Here's the drawing with two shaded views (mm, measured from the low corner). I have some questions. Give positions to 0.01 mm unless a question says otherwise; leave off trailing zeros. Write each loop counter-clockwise with the first axis right and the second up, starting at its lowest first coordinate (ties: lowest second). Pieces come first, ordered by that corner, then holes. Notation, with made-up numbers: (56, 31.5) - (98, 31.5) arc R21 cw to (98, 70.5) - close; hole circle Ø5 at (-34.5, 61.5). An arc over 180 degrees is marked (long way). Answer as a JSON object with one key per item and string values. Group by question number.
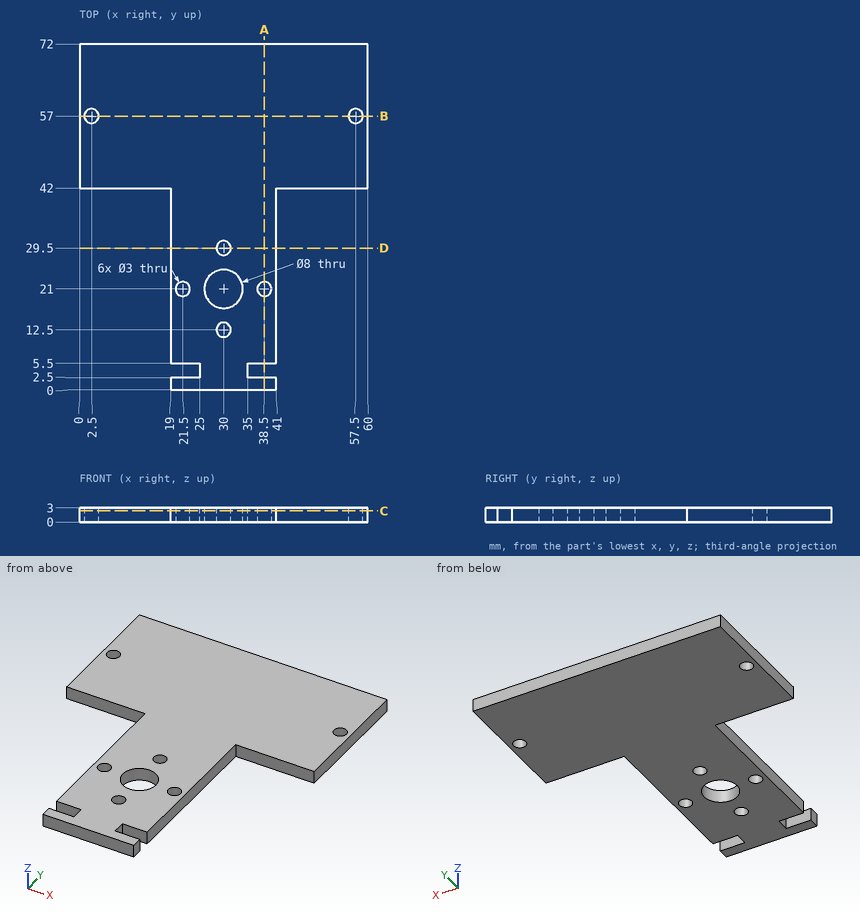
(1) I want a section at A-A, the plane x = 38.5. Please give me the cut outline in (y, z).
(2) I want a section at D-D, the plane y = 29.5. Please give me the cut outline in (x, z), and give its area (3 significant figures).
(3) I want a section at C-C, the plane z = 2.35. Please give me the cut outline in (x, y), and give its area (3 significant figures).
(4) Will these pins go through, and if not, where does the flat tip stop? P1, Ø9, axis at x = 30, y = 21, coming from the +Z side; P2, Ø1.5, axis at x = 13.5, z = 2, coming from the -Y side; P3, Ø0.9, axis at y = 22.5, z = 2, coming from the -X side; P4, Ø0.9, axis at y = 27, z = 2, coming from the +X side.
(5) I want a section at B-B, the plane y = 57. Please give me the cut outline in (x, z), and give its area (3 significant figures).
(6) I need wall thicknesses on L1, parallel to Y at x = 21.5, z = 1; L2, parallel to Y at x = 29, z = 1.9; L3, parallel to Y at x = 35.5, z = 0.75. Which ranges of each line are inside material? Lowest first, please.
Entries:
{
 "1": {"outline": "(0, 0) - (2.5, 0) - (2.5, 3) - (0, 3) - close; (5.5, 0) - (19.5, 0) - (19.5, 3) - (5.5, 3) - close; (22.5, 0) - (72, 0) - (72, 3) - (22.5, 3) - close"},
 "2": {"outline": "(19, 0) - (28.5, 0) - (28.5, 3) - (19, 3) - close; (31.5, 0) - (41, 0) - (41, 3) - (31.5, 3) - close", "area": "57.0 mm^2"},
 "3": {"outline": "(0, 42) - (19, 42) - (19, 5.5) - (25, 5.5) - (25, 2.5) - (19, 2.5) - (19, 0) - (41, 0) - (41, 2.5) - (35, 2.5) - (35, 5.5) - (41, 5.5) - (41, 42) - (60, 42) - (60, 72) - (0, 72) - close; hole circle Ø3 at (2.5, 57); hole circle Ø3 at (21.5, 21); hole circle Ø8 at (30, 21); hole circle Ø3 at (30, 12.5); hole circle Ø3 at (30, 29.5); hole circle Ø3 at (38.5, 21); hole circle Ø3 at (57.5, 57)", "area": "2,600 mm^2"},
 "4": {"P1": "z = 3", "P2": "y = 42", "P3": "x = 19", "P4": "x = 41"},
 "5": {"outline": "(0, 0) - (1, 0) - (1, 3) - (0, 3) - close; (4, 0) - (56, 0) - (56, 3) - (4, 3) - close; (59, 0) - (60, 0) - (60, 3) - (59, 3) - close", "area": "162 mm^2"},
 "6": {"L1": "0 to 2.5, 5.5 to 19.5, 22.5 to 72", "L2": "0 to 11.38, 13.62 to 17.13, 24.87 to 28.38, 30.62 to 72", "L3": "0 to 2.5, 5.5 to 72"}
}
